CAD build for the part. Positions are in the model's coordinates, mm. Coordinates: 2 decimals unless noted, no trailing zeros. Write each loop counter-clockwise with the first axis right and the second up, starting at its lowest first coordinate (ties: lowest second). Pieces come first, ordered by that corner, then holes. Notation, with made-up numbers: (-13.5, 48.5) - (13.5, 48.5) arc R23 ccw to (13.5, 72.5) - close; hole circle Ø10 at (84.25, 89.25). An arc over 180 degrees is marked (long way). Answer in a Markdown table with one row per item. Add a question column.
Q1. Band-saw the part on C-C (x = -2). List the corners of the cut face in (y, z) (3 decimals), and give its area (3 significant figures).
Q2. Drill centre lines: line 1 along Y through (x, z) = (0, 2.1); line 2 along Y through (x, z) = (-1, 1.1); line 3 along X through (y, z) = (1, 2.25). Where is each one in solid material? Low to high. Write a range as from..to.
Q3. Band-saw the part on A-A (x = 0). List the corners of the cut face in (y, z) (3 decimals).
Q4. Two-plate mould, pull along Y, no slides. Class faces 1 (the flat face through (0, 13, 0)), 2 (the cylindrical face through (-1.755, 27.009, 1.565)), 3 (the cylindrical face through (-0.08, -6.35, 1.57)): +Y half, -Y half, draft (parallel to the pull), parting line (faces both ways), or undercut.
Q5. Pin check, flat tips, straight feed: pin 1 (5.5 mm diameter, centred on x = 0, y = 25.4, fed in from -Z); pin 2 (4.5 mm diameter, centred on x = 0, y = 0, fed in from -Z). Stop position of each tip, or through.
Q6. Band-saw the part on B-B (z = 2.1). State how many separate pieces and enclosed holes the cut face has, and give its area (3 significant figures).
Q7. Band-saw the part on D-D (x = 4.5). List the corners of the cut face in (y, z) (3 decimals).
```python
from build123d import *

# Parameters (mm, degrees)
SKETCH1_R           = 2.38125
BOSS_EXTRUDE1_DEPTH = 3.175


with BuildPart() as part:
    # Sketch1 → Boss-Extrude1 (new body)
    with BuildSketch(Plane.XY):
        with BuildLine():
            ThreePointArc((5.995089754, 27.493179122), (0, 31.75), (-5.995089754, 27.493179122))
            add(Edge.make_bspline(
                [(-5.995089754, 27.493179122), (-6.695447175, 25.487280271), (-7.636062062, 20.832001378), (-5.83605341, 13.118062743), (-6.979750328, 4.623489499), (-7.03277938, -1.495925245), (-4.865611487, -4.080235883)],
                knots=[0, 0, 0, 0, 0.186998848, 0.456275956, 0.716521227, 1, 1, 1, 1], degree=3))
            ThreePointArc((-4.865611487, -4.080235883), (0, -6.35), (4.865611487, -4.080235883))
            add(Edge.make_bspline(
                [(5.995089754, 27.493179122), (6.695447175, 25.487280271), (7.636062062, 20.832001378), (5.83605341, 13.118062743), (6.979750328, 4.623489499), (7.03277938, -1.495925245), (4.865611487, -4.080235883)],
                knots=[0, 0, 0, 0, 0.186998848, 0.456275956, 0.716521227, 1, 1, 1, 1], degree=3))
        make_face()
        with Locations((0, 25.4)):
            Circle(SKETCH1_R, mode=Mode.SUBTRACT)
        Circle(SKETCH1_R, mode=Mode.SUBTRACT)
    extrude(amount=BOSS_EXTRUDE1_DEPTH)


solid = part.part
```
Checked values:
| question | item | result |
|---|---|---|
| 1 | outline | (-6.027, 0) - (-1.292, 0) - (-1.292, 3.175) - (-6.027, 3.175) - close; (1.292, 0) - (24.108, 0) - (24.108, 3.175) - (1.292, 3.175) - close; (26.692, 0) - (31.427, 0) - (31.427, 3.175) - (26.692, 3.175) - close |
| 1 | area | 103 mm² |
| 2 | line 1 | y = -6.35..-2.38, 2.38..23.02, 27.78..31.75 |
| 2 | line 2 | y = -6.27..-2.16, 2.16..23.24, 27.56..31.67 |
| 2 | line 3 | x = -6.82..-2.16, 2.16..6.82 |
| 3 | outline | (-6.35, 0) - (-2.381, 0) - (-2.381, 3.175) - (-6.35, 3.175) - close; (2.381, 0) - (23.019, 0) - (23.019, 3.175) - (2.381, 3.175) - close; (27.781, 0) - (31.75, 0) - (31.75, 3.175) - (27.781, 3.175) - close |
| 4 | face 1 | draft |
| 4 | face 2 | undercut |
| 4 | face 3 | -Y half |
| 5 | pin 1 | stops at z = 0 |
| 5 | pin 2 | passes through |
| 6 | separate pieces | 1 |
| 6 | enclosed holes | 2 |
| 6 | area | 434 mm² |
| 7 | outline | (-4.48, 0) - (29.88, 0) - (29.88, 3.175) - (-4.48, 3.175) - close |
